from build123d import *

# Parameters (mm, degrees)
F1_R     = 3.5
F1_R_2   = 1.5
F4_W     = 40
F4_H     = 13
F5_DEPTH = 20
F6_R     = 2.5
F7_DEPTH = 17.5
F8_R     = 2.5
F9_DEPTH = 13.7


with BuildPart() as f3:
    # F3: sweep along a path in F2
    with BuildLine(Plane.XZ) as f3_path:
        Line((-5.2793398216, 0), (-5.2793398216, -50))
        Line((-5.2793398216, -50), (-32.7452681959, -50))
        Line((-32.7452681959, -50), (-32.7452681959, -7.5485259295))
        Line((-32.7452681959, -7.5485259295), (-45.9185168147, -7.5485259295))
        Line((-45.9185168147, -7.5485259295), (-45.9185168147, -111.4290356636))
    # F1 (on Top) → F3 (sweep)
    with BuildSketch(Plane.XY):
        with Locations((-5.2793398216, -3.5)):
            Circle(F1_R)
        with Locations((-5.2793398216, -3.5)):
            Circle(F1_R_2, mode=Mode.SUBTRACT)
    sweep(path=f3_path.line, transition=Transition.RIGHT)

    # F4 (on face) → F5 (join)
    with BuildSketch(Plane.XZ):
        with Locations((-44.9899062514, -109.7345791803)):
            Rectangle(F4_W, F4_H)
    extrude(amount=F5_DEPTH)

    # F6 (on face) → F7 (cut)
    with BuildSketch(Plane(origin=(-64.9899062514, 0, 0), x_dir=(0, -1, 0), z_dir=(-1, 0, 0))):
        with Locations((2.9474398464, -112.3711525504)):
            Circle(F6_R)
    extrude(amount=-F7_DEPTH, mode=Mode.SUBTRACT)

    # F8 (on face) → F9 (cut)
    with BuildSketch(Plane(origin=(0, 0, -116.2345791803), x_dir=(1, 0, 0), z_dir=(0, 0, -1))):
        with Locations((-45.9672063589, 2.9437162448)):
            Circle(F8_R)
    extrude(amount=-F9_DEPTH, mode=Mode.SUBTRACT)


solid = f3.part
Geometry: final body of the model. Coordinates: model frame, mm. A direction names the side the tool comes from. Give positions to 0.01 mm unless a question says otherwise; leave off trailing zeros. Write each loop counter-clockwise with the first axis right and the second up, starting at its lowest first coordinate (ties: lowest second). Pieces come first, ordered by that corner, then holes. Notation, with made-up numbers: M 7,42.25 L 51,42.25 A23 cw 51,55.25 Z; hole C 50,65 d3. An arc over 180 degrees is marked long. Answer in a Markdown table with one row per item. Add a question column.
(1) First-contact query: pin 1 (4 mm diameter, centred on x = -45.97, y = -2.94, fed in from -Z); pin 2 (5 mm diameter, centred on x = -5.28, y = -3.5, fed in from -Z); pin 3 (2.5 mm diameter, centred on x = -32.75, y = -3.5, fed in from +Z). Flat tips, straight axial feed; report the tip coordinate or a pass-through.
(2) Ray query, line 1 (X direction, y = -3.75, z = -21); line 2 (Z direction, x = -51, y = -19); line 3 (Y direction, x = -45, z = -68). Return the intervals inside material, ascending.
(3) Reachability of faces 5 (the cylindrical face through (-2.046, -2.159, -27.124)), 6 (the cylindrical face through (-56.36, -4.1, -114.59)), 7 (the cylindrical face through (-19.25, -4.55, -53.34)), 8 (the flat face through (-45, -2, -102.535)) from +Z, -Z, +X, -X, +Y, -Y: full face, straight path, thin tool, end or side. Return the list, or none.
(4) Section C-C on x = -10.5. Return loops of the section in (y, z).
(5) Section A-A on z = -50. Return loops of the section in (x, y), and give its area (3 significant figures).
(6) Section B-B on z = -91. Return loops of the section in (x, y), and give its area (3 significant figures).
(7) Mould query, pull axis X, two halves, no side actions, for faces 1 (the flat face through (-45, 0, -110)), 2 (the cylindrical face through (-31.555, -2.587, -28.456)), 3 (the flat face through (-24.99, -10, -110)), 4 (the cylindrical face through (-19.23, -3.95, -51.43)). Classes: +X half, -X half, draft (parallel to the pull), parting line (faces both ways), or undercut.
(8) Section D-D on y = -15.75. Return loops of the section in (x, z), and give its area (3 significant figures).
Result set:
| question | item | result |
|---|---|---|
| 1 | pin 1 | stops at z = -102.53 |
| 1 | pin 2 | stops at z = -53.5 |
| 1 | pin 3 | stops at z = -4.05 |
| 2 | line 1 | x = -49.41 to -47.4, -44.44 to -42.43, -36.24 to -34.22, -31.27 to -29.25, -8.77 to -6.76, -3.8 to -1.79 |
| 2 | line 2 | z = -116.23 to -103.23 |
| 2 | line 3 | y = -6.88 to -4.69, -2.31 to -0.12 |
| 3 | face 5 | +Z |
| 3 | face 6 | -X |
| 3 | face 7 | none |
| 3 | face 8 | -Z |
| 4 | outline | C -3.5,-50 d7; hole C -3.5,-50 d3 |
| 5 | outline | C -45.92,-3.5 d7; M -32.75,-7 L -5.28,-7 A3.5 ccw -5.28,0 L -32.75,0 A3.5 ccw Z; hole C -45.92,-3.5 d3; hole M -32.75,-5 L -5.28,-5 A1.5 ccw -5.28,-2 L -32.75,-2 A1.5 ccw Z |
| 5 | area | 173 mm^2 |
| 6 | outline | C -45.92,-3.5 d7; hole C -45.92,-3.5 d3 |
| 6 | area | 31.4 mm^2 |
| 7 | face 1 | draft |
| 7 | face 2 | undercut |
| 7 | face 3 | +X half |
| 7 | face 4 | undercut |
| 8 | outline | M -64.99,-116.23 L -24.99,-116.23 L -24.99,-103.23 L -64.99,-103.23 Z |
| 8 | area | 520 mm^2 |
